Design review of the part built by this model. Coordinates are the model's own, in mm. A direction names the side the tool comes from. Give positions to 0.01 mm unless a question says otherwise; leave off trailing zeros. Order: outer loops, then holes, each group sorted by start corner. A loop starts at its lowest first (then second) coordinate and runs counter-clockwise, first axis right, second up. Notation, with made-up numbers: (-23, 61) - (7, 61) arc R15 ccw to (7, 80) - close; hole circle Ø11 at (49, -25.75). An arc over 180 degrees is marked (long way). Write each question's results on one line, items separated by ' | '. Start each with the question number.
```python
from build123d import *

# Parameters (mm, degrees)
BOSS_EXTRUDE1_DEPTH        = 10
CUT_EXTRUDE1_DEPTH         = 5
F_3_2_3_2_DIAMETER_HOLE1_D = 3.2
BOSS_EXTRUDE2_DEPTH        = 10
FILLET1_R                  = 3
FILLET2_R                  = 2
CUT_EXTRUDE6_DEPTH         = 2.5
SKETCH28_R                 = 3.5
CUT_EXTRUDE7_DEPTH         = 2.6
SKETCH29_W                 = 2.6
SKETCH29_H                 = 3.5
SKETCH30_R                 = 2.1
CUT_EXTRUDE8_DEPTH         = 6.829807515


with BuildPart() as part:
    # Sketch1 → Boss-Extrude1 (new body)
    with BuildSketch(Plane(origin=(0, 0, 0), x_dir=(1, 0, 0), z_dir=(0, 1, 0))):
        with BuildLine():
            ThreePointArc((-207.414551525, 32.851237658), (-210, 0), (-207.414551525, -32.851237658))
            Line((-207.414551525, -32.851237658), (-217.291434931, -34.415582309))
            ThreePointArc((-217.291434931, -34.415582309), (-220, 0), (-217.291434931, 34.415582309))
            Line((-217.291434931, 34.415582309), (-207.414551525, 32.851237658))
        make_face()
        with BuildLine():
            ThreePointArc((-217.291434931, -34.415582309), (-220, 0), (-217.291434931, 34.415582309))
            Line((-217.291434931, 34.415582309), (-220.254499953, 34.884885704))
            ThreePointArc((-220.254499953, 34.884885704), (-223, 0), (-220.254499953, -34.884885704))
            Line((-220.254499953, -34.884885704), (-217.291434931, -34.415582309))
        make_face()
        with BuildLine():
            Line((-204.451486503, 32.381934263), (-207.414551525, 32.851237658))
            ThreePointArc((-207.414551525, 32.851237658), (-210, 0), (-207.414551525, -32.851237658))
            Line((-207.414551525, -32.851237658), (-204.451486503, -32.381934263))
            ThreePointArc((-204.451486503, -32.381934263), (-207, 0), (-204.451486503, 32.381934263))
        make_face()
    extrude(amount=BOSS_EXTRUDE1_DEPTH)

    # Sketch15 → Cut-Extrude1 (cut)
    with BuildSketch(Plane(origin=(0, 10, 0), x_dir=(1, 0, 0), z_dir=(0, 1, 0))):
        with BuildLine():
            Line((-219.772609758, 10), (-209.761769634, 10))
            ThreePointArc((-209.761769634, 10), (-208.900850883, 21.457737542), (-207.414551525, 32.851237658))
            Line((-207.414551525, 32.851237658), (-217.291434931, 34.415582309))
            ThreePointArc((-217.291434931, 34.415582309), (-218.872736893, 22.242415451), (-219.772609758, 10))
        make_face()
        with BuildLine():
            ThreePointArc((-207.414551525, -32.851237658), (-208.900850883, -21.457737542), (-209.761769634, -10))
            Line((-209.761769634, -10), (-219.772609758, -10))
            ThreePointArc((-219.772609758, -10), (-218.872736893, -22.242415451), (-217.291434931, -34.415582309))
            Line((-217.291434931, -34.415582309), (-207.414551525, -32.851237658))
        make_face()
    extrude(amount=-CUT_EXTRUDE1_DEPTH, mode=Mode.SUBTRACT)

    # Ø3.2 (3.2) Diameter Hole1 (through all)
    with Locations(Plane(origin=(0, 0, 0), x_dir=(-1, 0, 0), z_dir=(0, -1, 0))):
        with Locations((214.18186009, -18.738484691), (214.18186009, 18.738484691)):
            Hole(F_3_2_3_2_DIAMETER_HOLE1_D / 2)

    # Sketch19 → Boss-Extrude2 (add)
    with BuildSketch(Plane(origin=(0, 0, 0), x_dir=(1, 0, 0), z_dir=(0, 1, 0))):
        with BuildLine():
            Line((-205.060008726, -13.440343057), (-206.55679711, -13.538447751))
            ThreePointArc((-206.55679711, -13.538447751), (-207, 0), (-206.55679711, 13.538447751))
            Line((-206.55679711, 13.538447751), (-205.060008726, 13.440343057))
            ThreePointArc((-205.060008726, 13.440343057), (-205.5, 0), (-205.060008726, -13.440343057))
        make_face()
    extrude(amount=BOSS_EXTRUDE2_DEPTH)

    # Fillet1
    # the kernel refuses this fillet: 3 mm, written as the material it adds along each edge
    with BuildSketch(Plane(origin=(-206.55679711, 0, -13.538447751), x_dir=(0.071732779716433, 0, -0.9974238859753429), z_dir=(0, 1, 0))) as fillet1_piece_1:
        with BuildLine():
            CenterArc((2.607610468, -2.999939619), FILLET1_R, 89.636481565, 60.364184224)
            Line((0.009516827, -1.49996981), (-0.042445046, -1.469970414))
            ThreePointArc((-0.042445046, -1.469970414), (-0.055240379, -0.750365578), (-0.059998792, -0.000380673))
            Line((-0.059998792, -0.000380673), (-0.000380673, 0.059998792))
            ThreePointArc((-0.000380673, 0.059998792), (1.313322061, 0.064166261), (2.627024794, 0.059998792))
            Line((2.627024794, 0.059998792), (2.626644121, 0))
        make_face()
    extrude(amount=10)
    with BuildSketch(Plane(origin=(-206.55679711, 0, 13.538447751), x_dir=(0.07173277971643319, 0, 0.9974238859753429), z_dir=(0, 1, 0))) as fillet1_piece_2:
        with BuildLine():
            CenterArc((2.607610468, 2.999939619), FILLET1_R, 209.999334211, 60.364184224)
            Line((0.009516827, 1.49996981), (-0.042445046, 1.469970414))
            ThreePointArc((-0.042445046, 1.469970414), (-0.055240379, 0.750365578), (-0.059998792, 0.000380673))
            Line((-0.059998792, 0.000380673), (-0.000380673, -0.059998792))
            ThreePointArc((-0.000380673, -0.059998792), (1.313322061, -0.064166261), (2.627024794, -0.059998792))
            Line((2.627024794, -0.059998792), (2.626644121, 0))
        make_face()
    extrude(amount=10)

    # Fillet2
    fillet2_edges = [part.edges().sort_by_distance(p)[0] for p in [
        (-220.254499953, 5, 34.884885704),
        (-220.254499953, 5, -34.884885704),
        (-204.451486503, 5, -32.381934263),
        (-204.451486503, 5, 32.381934263),
    ]]
    fillet(fillet2_edges, radius=FILLET2_R)

    # Sketch26 → Cut-Extrude6 (cut)
    with BuildSketch(Plane.XZ):
        with BuildLine():
            Line((-218.270184732, -34.570601048), (-206.417411405, -32.693306179))
            ThreePointArc((-206.417411405, -32.693306179), (-205.117889671, -31.901228423), (-204.75200014, -30.423978019))
            ThreePointArc((-204.75200014, -30.423978019), (-205.683905744, -23.30516934), (-206.368380626, -16.158325337))
            ThreePointArc((-206.368380626, -16.158325337), (-206.080650798, -14.622930952), (-205.060008726, -13.440343057))
            ThreePointArc((-205.060008726, -13.440343057), (-205.5, 0), (-205.060008726, 13.440343057))
            ThreePointArc((-205.060008726, 13.440343057), (-206.080650798, 14.622930952), (-206.368380626, 16.158325337))
            ThreePointArc((-206.368380626, 16.158325337), (-205.683905744, 23.30516934), (-204.75200014, 30.423978019))
            ThreePointArc((-204.75200014, 30.423978019), (-205.117889671, 31.901228423), (-206.417411405, 32.693306179))
            Line((-206.417411405, 32.693306179), (-218.270184732, 34.570601048))
            ThreePointArc((-218.270184732, 34.570601048), (-219.765933628, 34.207922413), (-220.561180845, 32.890203773))
            ThreePointArc((-220.561180845, 32.890203773), (-223, 0), (-220.561180845, -32.890203773))
            ThreePointArc((-220.561180845, -32.890203773), (-219.765933628, -34.207922413), (-218.270184732, -34.570601048))
        make_face()
    extrude(amount=-CUT_EXTRUDE6_DEPTH, mode=Mode.SUBTRACT)

    # Sketch28 → Cut-Extrude7 (cut)
    with BuildSketch(Plane(origin=(-217.5, 0, 0), x_dir=(0, 0, -1), z_dir=(1, 0, 0))):
        with Locations((0, 10)):
            Circle(SKETCH28_R)
    extrude(amount=CUT_EXTRUDE7_DEPTH, mode=Mode.SUBTRACT)

    # Sketch29 → Cut-Revolve1 (revolve, cut)
    with BuildSketch(Plane(origin=(0, 10, 0), x_dir=(1, 0, 0), z_dir=(0, 1, 0))):
        with Locations((-206.770192485, -1.75)):
            Rectangle(SKETCH29_W, SKETCH29_H)
    revolve(axis=Axis((-217.5, 10, 0), (1, 0, 0)), mode=Mode.SUBTRACT)

    # Sketch30 → Cut-Extrude8 (cut)
    with BuildSketch(Plane(origin=(-208.070192485, 0, 0), x_dir=(0, 0, -1), z_dir=(1, 0, 0))):
        with Locations((0, 10)):
            Circle(SKETCH30_R)
    extrude(amount=-CUT_EXTRUDE8_DEPTH, mode=Mode.SUBTRACT)


solid = part.part
```
Q1. Add section C-C (y = 3.25). Give the boundary of the cut face in (x, z).
Q2. Add section B-B (y = 7.25). Give the boundary of the cut face in (x, z).
Q3. Add section A-A (z = 0). Give the boundary of the cut face in (x, y).
Q4. Insertion check: pin 1 Ø3 at (y, z) = (9, -1.5) entering from -X; pin 2 Ø4 at (y, z) = (8, 23.5) entering from +X; pin 3 Ø4 at (y, z) = (9, -0.5) entering from +X; pin 4 Ø3.5 at (x, z) = (-213, 25.5) entering from +Y. Each pin has a flat end and moves straight along its axis. Give the tip position at first contact, or say it passes through.
Q5. Machinability: for faces 4 (the cylindrical face through (-206.8, 6.5, 0.1)), 5 (the cylindrical face through (-206.09, 6.2, -14.64)), 6 (the cylindrical face through (-208.917, 7.535, -21.298)), 7 (the cylindrical face through (-216.2, 6.5, 0.1)), which of the approach directions +Z, -Z, +X, -X, +Y, -Y give a long, thin tool a straight path to every point of the face, cutting with its end or side? Answer none if there is none.
Q6. Draft analysis for pull direction Z (two halves, no side actions). For faces 1 (the cylindrical face through (-215.45, 3.77, -17.76)), 2 (the cylindrical face through (-219.75, 6.3, -34.22)), 3 (the flat face through (-214, 2.5, 0)), state which applies: pulls with the +Z half, pulls with the -Z half, needs draft (parallel to the pull), parting line crosses it, or undercut.
Q7. For line 1 (Z direction, x = -215, y = 4.75); line 2 (X direction, y = 7, z = -0.5); line 3 (Z direction, x = -214, y = 9.75), list the stretches that pass through material, from the lowest coordinate up. Write a range as [from, to].
Verdict:
1) outline: (-220.56, -32.89) arc R2 ccw to (-218.27, -34.57) - (-206.42, -32.69) arc R2 ccw to (-204.75, -30.42) arc R207 cw to (-206.37, -16.16) arc R3 cw to (-205.06, -13.44) arc R205.5 cw to (-205.06, 13.44) arc R3 cw to (-206.37, 16.16) arc R207 cw to (-204.75, 30.42) arc R2 ccw to (-206.42, 32.69) - (-218.27, 34.57) arc R2 ccw to (-220.56, 32.89) arc R223 ccw to start; hole circle Ø3.2 at (-214.18, -18.74); hole circle Ø3.2 at (-214.18, 18.74)
2) outline: (-220.56, -32.89) arc R2 ccw to (-218.27, -34.57) - (-217.29, -34.42) arc R220 cw to (-219.77, -10) - (-209.76, -10) arc R210 ccw to (-207.41, -32.85) - (-206.42, -32.69) arc R2 ccw to (-204.75, -30.42) arc R207 cw to (-206.37, -16.16) arc R3 cw to (-205.06, -13.44) arc R205.5 cw to (-205.49, -2.17) - (-208.07, -2.17) - (-208.07, 2.17) - (-205.49, 2.17) arc R205.5 cw to (-205.06, 13.44) arc R3 cw to (-206.37, 16.16) arc R207 cw to (-204.75, 30.42) arc R2 ccw to (-206.42, 32.69) - (-207.41, 32.85) arc R210 ccw to (-209.76, 10) - (-219.77, 10) arc R220 cw to (-217.29, 34.42) - (-218.27, 34.57) arc R2 ccw to (-220.56, 32.89) arc R223 ccw to start; hole (-217.5, -2.17) - (-214.9, -2.17) - (-214.9, 2.17) - (-217.5, 2.17) - close
3) outline: (-223, 2.5) - (-205.5, 2.5) - (-205.5, 6.5) - (-208.07, 6.5) - (-208.07, 7.9) - (-214.9, 7.9) - (-214.9, 6.5) - (-217.5, 6.5) - (-217.5, 10) - (-223, 10) - close
4) pin 1: stops at x = -223 | pin 2: stops at x = -205.42 | pin 3: stops at x = -208.07 | pin 4: stops at y = 5
5) face 4: +X, +Y | face 5: +X, +Y, -Y | face 6: -Z, +Y | face 7: +Y
6) face 1: undercut | face 2: pulls with the -Z half | face 3: needs draft
7) line 1: z = [-34.05, -20.11], [-17.36, 17.36], [20.11, 34.05] | line 2: x = [-223, -217.5], [-214.9, -208.07] | line 3: z = [-10, -2.09], [2.09, 10]
